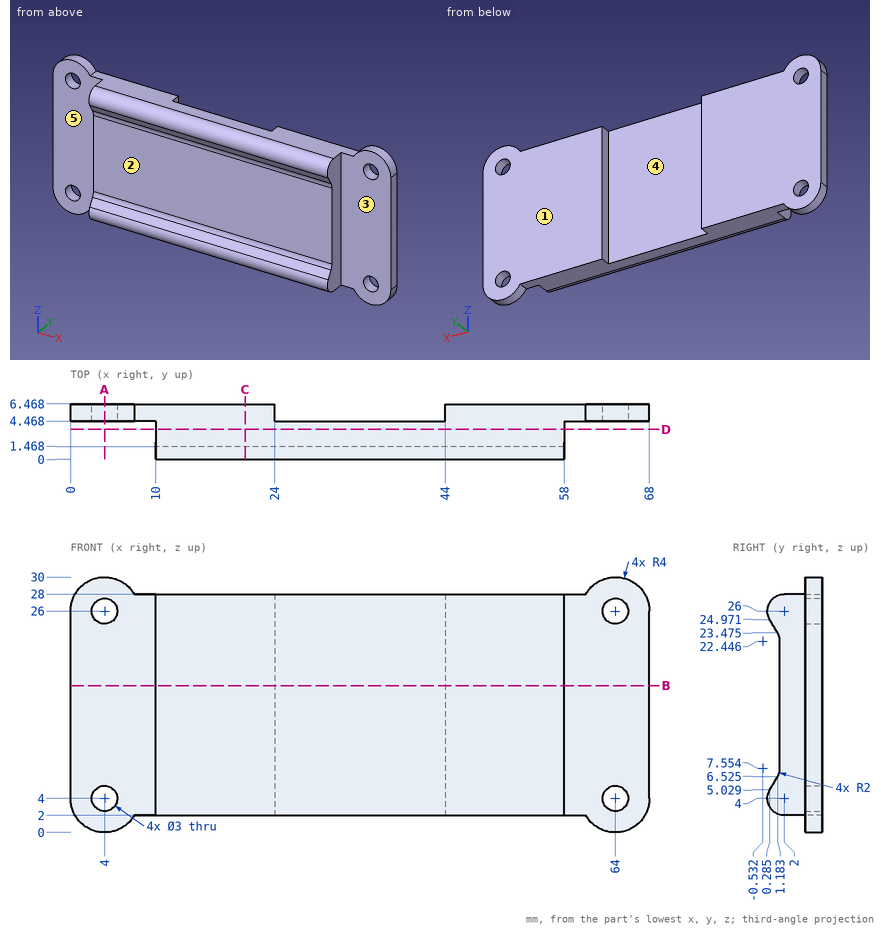
Print and shaded views of the part. All mm, measured from the part's lowest x, y and z. A direction names the side the tool comes from. Give positions to 0.01 mm unless a question says otherwise; leave off trailing zeros. Write each loop counter-clockwise with the first axis right and the second up, starting at its lowest first coordinate (ties: lowest second). Pieces come first, ordered by that corner, then holes. Notation, with made-up numbers: (60.25, -21.5) - (101.25, -21.5) arc R23 ccw to (101.25, -11.5) - close; hole circle Ø4 at (58.5, -19.75). An arc over 180 degrees is marked (long way). Put each result on its own line as item: value.
(1) Tool access for the marked faces 1, 2 and 3: list every direction of +Z, -Z, +X, -X, +Y, -Y with a clear straight run to the whole face (end or side of a thin tool).
Working result:
face 1: +Z, -Z, +X, -X, +Y
face 2: +X, -X, -Y
face 3: +Z, -Z, +X, -Y
(2) Drop flat-ended pins along their axis: pin 1 Ø1.3 at (x, y) = (27.5, 5) entering from +Z; pin 2 Ø1.3 at (y, z) = (2.5, 15) entering from -X; pin 3 Ø2 at (x, z) = (7, 6.5) entering from -Y. Give the stop position or say it passes through.
Working result:
pin 1: z = 28
pin 2: x = 10
pin 3: y = 4.47
(3) Saw through at C-C (x = 20.5). List the corners of the cut face in (y, z) (1 decimal), then the cut area to 3 significant figures.
Working result:
outline: (0.3, 5) arc R2 ccw to (2, 2) - (6.5, 2) - (6.5, 28) - (2, 28) arc R2 ccw to (0.3, 25) - (1.2, 23.5) arc R2 cw to (1.5, 22.4) - (1.5, 7.6) arc R2 cw to (1.2, 6.5) - close
area: 139 mm^2
(4) Saw through at D-D (y = 3.5). List the corners of the cut face in (x, z).
Working result:
outline: (10, 2) - (58, 2) - (58, 28) - (10, 28) - close
(5) Saw through at A-A (x = 4). List the corners of the cut face in (y, z), then the cut area to 3 significant figures.
Working result:
outline: (4.47, 0) - (6.47, 0) - (6.47, 2.5) - (4.47, 2.5) - close; (4.47, 5.5) - (6.47, 5.5) - (6.47, 24.5) - (4.47, 24.5) - close; (4.47, 27.5) - (6.47, 27.5) - (6.47, 30) - (4.47, 30) - close
area: 48.0 mm^2
(6) Saw through at B-B (z = 17.25). List the corners of the cut face in (x, y).
Working result:
outline: (0, 4.47) - (10, 4.47) - (10, 1.47) - (58, 1.47) - (58, 4.47) - (68, 4.47) - (68, 6.47) - (44, 6.47) - (44, 4.47) - (24, 4.47) - (24, 6.47) - (0, 6.47) - close
(7) Pull direction X, two halves, no side cores. Call the marked faces 4 and 5: released by +X, released by -X, zero draft, split by the parting line, or undercut.
Working result:
face 4: undercut
face 5: zero draft
(8) Wall check: L1, parallel to X at y = 5.2, z = 26; L2, parallel to Z at x = 64, y = 5.25; L3, parallel to X at y = 6.25, z = 21.5. Give the ranges that are in metal, low to high.
Working result:
L1: 0 to 2.5, 5.5 to 24, 44 to 62.5, 65.5 to 68
L2: 0 to 2.5, 5.5 to 24.5, 27.5 to 30
L3: 0 to 24, 44 to 68
